Can you work these out from the model? Positions are in its coordinate system, mm. A direction names the side the tool comes from. Give positions to 0.01 mm unless a question says otherwise; leave off trailing zeros. Order: outer loops, then holes, each group sorted by start corner. A loop starts at its lowest first (then second) coordinate and runs counter-clockwise, first axis right, second up. Notation, with made-up numbers: (72, 67.25) -> (76, 67.25) arc R14 cw to (76, 92.25) -> close; hole circle Ø8 at (29, -18). An arc over 180 degrees is marked (long way). Answer as a JSON object with one key per item and string values.
```python
from build123d import *

# Parameters (mm, degrees)
F1_DEPTH = 50
F2_R     = 10.899508
F3_DEPTH = 25
F4_SIZE  = 5


with BuildPart() as f1:
    # F0 (on Top) → F1 (new body)
    with BuildSketch(Plane.XY):
        with BuildLine():
            Line((-35.020374, 9.075959), (-35.020374, -24.844296))
            Line((-35.020374, -24.844296), (23.102446, -24.844296))
            Line((23.102446, -24.844296), (23.102446, -17.734874))
            ThreePointArc((23.102446, -17.734874), (2.064421, -12.059264), (-3.237784, 9.075959))
            Line((-3.237784, 9.075959), (-35.020374, 9.075959))
        make_face()
        with BuildLine():
            Line((23.102446, 9.075959), (23.102446, -17.734874))
            ThreePointArc((23.102446, -17.734874), (34.530424, -10.031296), (38.942748, 3.02532))
            ThreePointArc((38.942748, 3.02532), (20.474798, 24.331467), (-3.237784, 9.075959))
            Line((-3.237784, 9.075959), (23.102446, 9.075959))
        make_face()
        with BuildLine():
            ThreePointArc((-3.237784, 9.075959), (2.064421, -12.059264), (23.102446, -17.734874))
            Line((23.102446, -17.734874), (23.102446, 9.075959))
            Line((23.102446, 9.075959), (-3.237784, 9.075959))
        make_face()
    extrude(amount=F1_DEPTH)

    # F2 (on face) → F3 (join)
    with BuildSketch(Plane(origin=(-35.020374, 0, 0), x_dir=(0, -1, 0), z_dir=(-1, 0, 0))):
        with Locations((8.835716, 25.147455)):
            Circle(F2_R)
    extrude(amount=F3_DEPTH)

    # F4
    f4_edges = [f1.edges().sort_by_distance(p)[0] for p in [
        (23.102446, -24.844296, 25),
        (-35.020374, -24.844296, 25),
        (-5.958964, -24.844296, 0),
        (-5.958964, -24.844296, 50),
    ]]
    chamfer(f4_edges, length=F4_SIZE)


solid = f1.part
```
1. For faces 1 (the face through (-47.345, -14.695, 34.338)), 2 (the face through (-32.485, -22.379, 24.65)), 3 (the face through (23.102, -19, 25)), 4 (the face through (-19, 9.076, 25)), which set-ups out of +Z, -Z, +X, -X, +Y, -Y let a thin tool reach every point of the face, with its end or its side?
Worked answers:
{"face 1": "-X", "face 2": "+Z, -Z, -X, -Y", "face 3": "+Z, -Z, +X, -Y", "face 4": "+Z, -Z, -X, +Y"}
2. If we section it at C-C on y = -2: Please give me the cut outline in (x, z).
Worked answers:
{"outline": "(-60.02, 16.66) -> (-35.02, 16.66) -> (-35.02, 0) -> (38.35, 0) -> (38.35, 50) -> (-35.02, 50) -> (-35.02, 33.64) -> (-60.02, 33.64) -> close"}
3. If we section it at D-D on z = 17.5: Please give me the cut outline in (x, y).
Worked answers:
{"outline": "(-60.02, -16.6) -> (-35.02, -16.6) -> (-35.02, -19.84) -> (-30.02, -24.84) -> (18.1, -24.84) -> (23.1, -19.84) -> (23.1, -17.73) arc R21.52 ccw to (38.94, 3.03) arc R21.52 ccw to (-3.24, 9.08) -> (-35.02, 9.08) -> (-35.02, -1.07) -> (-60.02, -1.07) -> close"}
4. If we section it at B-B on x = -21: Please give me the cut outline in (y, z).
Worked answers:
{"outline": "(-24.84, 5) -> (-19.84, 0) -> (9.08, 0) -> (9.08, 50) -> (-19.84, 50) -> (-24.84, 45) -> close"}
5. Will these pins go through, and if not, where does the flat tip stop? pin 1 Ø0.6 at (y, z) = (-19, 14.5) entering from +X; pin 2 Ø10 at (y, z) = (-14.5, 8) entering from -X; pin 3 Ø5 at (x, y) = (-5.5, 13) entering from +Z; pin 4 Ø8 at (y, z) = (18, 9) entering from +X.
Worked answers:
{"pin 1": "x = 23.1", "pin 2": "x = -35.02", "pin 3": "through", "pin 4": "x = 35.93"}
6. If we section it at A-A on z = 40: Please give me the cut outline in (x, y), then the cut area to 3 significant figures.
Worked answers:
{"outline": "(-35.02, -19.84) -> (-30.02, -24.84) -> (18.1, -24.84) -> (23.1, -19.84) -> (23.1, -17.73) arc R21.52 ccw to (38.94, 3.03) arc R21.52 ccw to (-3.24, 9.08) -> (-35.02, 9.08) -> close", "area": "2,750 mm²"}
7. Please list where these lines run through material, in increasing order: L1, parallel to Y at x = -29, z = 18; L2, parallel to Y at x = 18, z = 26.5; L3, parallel to X at y = -18.5, z = 10.
Worked answers:
{"L1": "-24.84 to 9.08", "L2": "-24.84 to 24.54", "L3": "-35.02 to 23.1"}
